Answer from the drawing. Dimensions are ordinates in mm from the lowest x, y and z of the part. A direction names the side the tool comes from. Give positions to 0.01 mm unless a question says otherwise; leave off trailing zeros. Write each loop counter-clockwise with the first axis right and the second up, starting at its lowest first coordinate (ties: lowest second). Pieces come first, ordered by that corner, then holes.
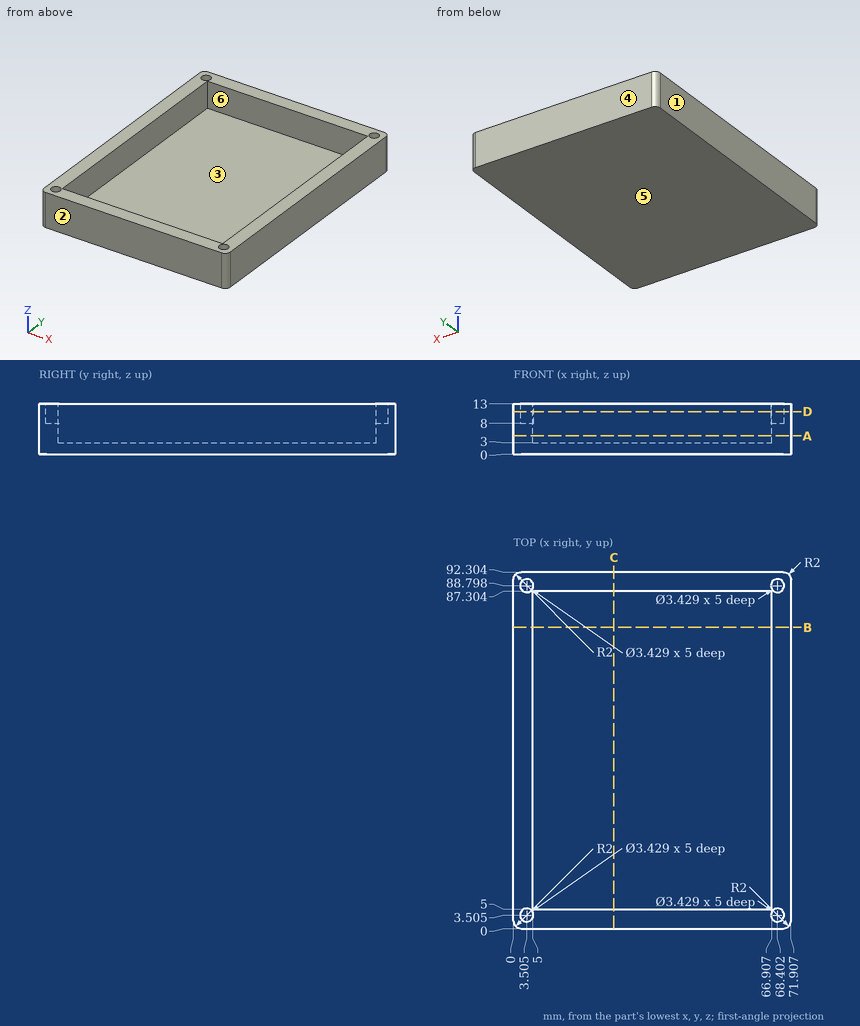
Item 1: Which of the six approach directions +Z, -Z, +X, -X, +Y, -Y give full straight-line access (tool end or side, diameter ignored) to the marked faces 5 and 6?
Result set:
face 5: -Z, +X, -X, +Y, -Y
face 6: +Z
Item 2: Section B-B (y = 78) is taken. Write down the section's boundary in (x, z).
Result set:
outline: (0, 0) - (71.91, 0) - (71.91, 13) - (66.91, 13) - (66.91, 3) - (5, 3) - (5, 13) - (0, 13) - close
Item 3: Each of these flat-tipped pins is pushed along its axis until it touches: pin 1 Ø8 at (x, y) = (58.5, 24) entering from +Z; pin 2 Ø3 at (x, y) = (68.4, 3.51) entering from +Z. Where does it stop, or does it pass through?
Result set:
pin 1: stops at z = 3
pin 2: stops at z = 8
Item 4: Determine the mould class of the marked faces 1, 2, 3 and 4 for opening direction Y: pulls with the +Y half, pulls with the -Y half, needs draft (parallel to the pull), parting line crosses it, or undercut.
Result set:
face 1: needs draft
face 2: pulls with the -Y half
face 3: undercut
face 4: pulls with the +Y half
Item 5: Find the intervals of material crossed by line 1 along X through (y, z) = (82, 10); line 2 along Y through (x, z) = (26.5, 7); line 3 along Z through (x, y) = (55, 48.5), in increasing order.
Result set:
line 1: x = 0 to 5, 66.91 to 71.91
line 2: y = 0 to 5, 87.3 to 92.3
line 3: z = 0 to 3
Item 6: Section A-A (z = 4.75) is taken. Write down the section's boundary in (x, y).
Result set:
outline: (0, 2) arc R2 ccw to (2, 0) - (69.91, 0) arc R2 ccw to (71.91, 2) - (71.91, 90.3) arc R2 ccw to (69.91, 92.3) - (2, 92.3) arc R2 ccw to (0, 90.3) - close; hole (5, 5) - (66.91, 5) - (66.91, 87.3) - (5, 87.3) - close
Item 7: Section D-D (z = 11) is taken. Write down the section's boundary in (x, y) (1 decimal).
Result set:
outline: (0, 2) arc R2 ccw to (2, 0) - (69.9, 0) arc R2 ccw to (71.9, 2) - (71.9, 90.3) arc R2 ccw to (69.9, 92.3) - (2, 92.3) arc R2 ccw to (0, 90.3) - close; hole circle Ø3.4 at (3.5, 3.5); hole circle Ø3.4 at (3.5, 88.8); hole (5, 5) - (66.9, 5) - (66.9, 87.3) - (5, 87.3) - close; hole circle Ø3.4 at (68.4, 3.5); hole circle Ø3.4 at (68.4, 88.8)
Item 8: Section C-C (x = 26) is taken. Write down the section's boundary in (y, z), and give its area (3 significant figures).
Result set:
outline: (0, 0) - (92.3, 0) - (92.3, 13) - (87.3, 13) - (87.3, 3) - (5, 3) - (5, 13) - (0, 13) - close
area: 377 mm2
